Verification items for the finished model (mm, model axes). Face numbers are marked on the shaded views. A direction names the side the tool comes from. Coordinates: 2 decimals unless noted, no trailing zeros. Order: outer loops, then holes, each group sorted by start corner. A loop starts at its lowest first (then second) coordinate and runs counter-clockwise, first axis right, second up. Notation, with made-up numbers: (88, 0) -> (143, 0) arc R20 cw to (143, 29) -> close; hole circle Ø6 at (-38.5, 63.25). An arc over 180 degrees is marked (long way). Write each question's results on one line, items separated by ' | '. Start each with the question number.
(1) Cross-section at A-A on x = -2.5. Enter the section's corners in (y, z), and give its area (3 significant figures).
(2) Thickness scan on probe 1 along Y at (x, z) = (-3, -10); probe 2 along Y at (x, z) = (9.5, 3); probe 3 along Z at (x, y) = (1, 13.5). Record the ranges inside material, lowest first. Write a range as [from, to].
(3) Go/stop test with flat-tipped pins: pin 1 (7 mm diameter, centred on x = 0, y = 7.5, fed in from -Z); pin 2 (6 mm diameter, centred on x = 11, z = 12, fed in from +Y); pin 3 (3 mm diameter, centred on x = -8.01, z = 13.94, fed in from +Y); pin 4 (10 mm diameter, centred on y = 10.5, z = 3.19, fed in from +X) (1 decimal). Record where each tip stops, or that it passes through.
(4) Cross-section at C-C on x = -8.5. Enter the section's corners in (y, z).
(5) Set-up check for the marked faces 1, 2 and 3: record each of +Z, -Z, +X, -X, +Y, -Y from which the full face is reachable in a straight line by a thin tool's end or side.
(6) Draft check along Y on the marked faces 4, 5 and 6. Enter one of: +Y half, -Y half, draft (parallel to the pull), parting line (faces both ways), or undercut.
(7) Cross-section at B-B on y = 14. Enter the section's corners in (x, z).
(8) Cross-section at D-D on z = 0. Enter the section's corners in (x, y), and give its area (3 significant figures).
```python
from build123d import *

# Parameters (mm, degrees)
SKETCH1_W            = 27
SKETCH1_H            = 35
SKETCH1_R            = 1.113712744
SKETCH1_R_2          = 1.000106258
SKETCH1_R_3          = 1.174626552
SKETCH1_R_4          = 1.19920455
SKETCH1_W_2          = 8.3
SKETCH1_H_2          = 2.12
BOSS_EXTRUDE1_DEPTH  = 2
M2_CLEARANCE_HOLE2_D = 2.4
SKETCH13_W           = 27
SKETCH13_H           = 17
BOSS_EXTRUDE6_DEPTH  = 17
SKETCH14_R           = 6.4
CUT_EXTRUDE3_DEPTH   = 38.815687555


with BuildPart() as part:
    # Sketch1 → Boss-Extrude1 (new body)
    # profile 1 of 8: a face of its own
    with BuildSketch(Plane(origin=(0, 0, 0), x_dir=(1, 0, 0), z_dir=(0, 1, 0))):
        with Locations((0.988085162, -0.939800033)):
            Rectangle(SKETCH1_W, SKETCH1_H)
        Polygon((-10.011914838, -15.939800033), (-10.011914838, 14.060199967), (11.988085162, 14.060199967), (11.988085162, -15.939800033), (5.138085162, -15.939800033), (5.138085162, -18.059800033), (-3.161914838, -18.059800033), (-3.161914838, -15.939800033), align=None, mode=Mode.SUBTRACT)
    # profile 2 of 8: a face of its own
    with BuildSketch(Plane(origin=(0, 0, 0), x_dir=(1, 0, 0), z_dir=(0, 1, 0))):
        Polygon((11.988085162, 14.060199967), (-10.011914838, 14.060199967), (-10.011914838, -15.939800033), (-3.161914838, -15.939800033), (-3.161914838, -13.819800033), (5.138085162, -13.819800033), (5.138085162, -15.939800033), (11.988085162, -15.939800033), align=None)
        with Locations((-8.011914838, -13.939800033)):
            Circle(SKETCH1_R, mode=Mode.SUBTRACT)
        with Locations((9.988085162, -14.291814947)):
            Circle(SKETCH1_R_2, mode=Mode.SUBTRACT)
        with Locations((-8.011914838, 7.560199967)):
            Circle(SKETCH1_R_3, mode=Mode.SUBTRACT)
        with Locations((9.988085162, 7.560199967)):
            Circle(SKETCH1_R_4, mode=Mode.SUBTRACT)
    # profile 3 of 8: a face of its own
    with BuildSketch(Plane(origin=(0, 0, 0), x_dir=(1, 0, 0), z_dir=(0, 1, 0))):
        with Locations((-8.011914838, 7.560199967)):
            Circle(SKETCH1_R_3)
    # profile 4 of 8: a face of its own
    with BuildSketch(Plane(origin=(0, 0, 0), x_dir=(1, 0, 0), z_dir=(0, 1, 0))):
        with Locations((9.988085162, 7.560199967)):
            Circle(SKETCH1_R_4)
    # profile 5 of 8: a face of its own
    with BuildSketch(Plane(origin=(0, 0, 0), x_dir=(1, 0, 0), z_dir=(0, 1, 0))):
        with Locations((9.988085162, -14.291814947)):
            Circle(SKETCH1_R_2)
    # profile 6 of 8: a face of its own
    with BuildSketch(Plane(origin=(0, 0, 0), x_dir=(1, 0, 0), z_dir=(0, 1, 0))):
        with Locations((0.988085162, -16.999800033)):
            Rectangle(SKETCH1_W_2, SKETCH1_H_2)
    # profile 7 of 8: a face of its own
    with BuildSketch(Plane(origin=(0, 0, 0), x_dir=(1, 0, 0), z_dir=(0, 1, 0))):
        with Locations((0.988085162, -14.879800033)):
            Rectangle(SKETCH1_W_2, SKETCH1_H_2)
    # profile 8 of 8: a face of its own
    with BuildSketch(Plane(origin=(0, 0, 0), x_dir=(1, 0, 0), z_dir=(0, 1, 0))):
        with Locations((-8.011914838, -13.939800033)):
            Circle(SKETCH1_R)
    extrude(amount=BOSS_EXTRUDE1_DEPTH)

    # M2 Clearance Hole2 (through all)
    with Locations(Plane(origin=(0, 2, 0), x_dir=(1, 0, 0), z_dir=(0, 1, 0))):
        with Locations((-8.011914838, 7.560199967), (9.988085162, 7.560199967), (-8.011914838, -13.939800033), (9.988085162, -14.291814947)):
            Hole(M2_CLEARANCE_HOLE2_D / 2)

    # Sketch13 → Boss-Extrude6 (add)
    with BuildSketch(Plane(origin=(0, 2, 0), x_dir=(1, 0, 0), z_dir=(0, 1, 0))):
        with Locations((0.988085162, -3.189800033)):
            Rectangle(SKETCH13_W, SKETCH13_H)
    extrude(amount=BOSS_EXTRUDE6_DEPTH)

    # Sketch14 → Cut-Extrude3 (cut, through all)
    with BuildSketch(Plane(origin=(14.488085162, 0, 0), x_dir=(0, 0, -1), z_dir=(1, 0, 0))):
        with Locations((-3.189800033, 10.5)):
            Circle(SKETCH14_R)
        with BuildLine():
            Line((5.310199967, 19), (-3.189800009, 19))
            ThreePointArc((-3.189800009, 19), (2.820607616, 16.510407631), (5.310199967, 10.5))
            Line((5.310199967, 10.5), (5.310199967, 19))
        make_face()
        with BuildLine():
            Line((-3.189800009, 19), (-11.689800033, 19))
            Line((-11.689800033, 19), (-11.689800033, 10.50000002))
            ThreePointArc((-11.689800033, 10.50000002), (-9.200207658, 16.510407656), (-3.189800009, 19))
        make_face()
    extrude(amount=-CUT_EXTRUDE3_DEPTH, mode=Mode.SUBTRACT)


solid = part.part
```
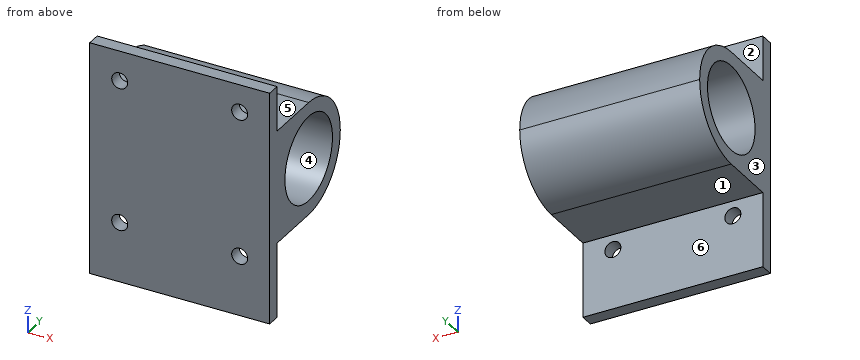
Results are:
1) outline: (0, -16.56) -> (2, -16.56) -> (2, -5.31) -> (10.5, -5.31) arc R8.5 ccw to (10.5, 11.69) -> (2, 11.69) -> (2, 18.44) -> (0, 18.44) -> close; hole circle Ø12.8 at (10.5, 3.19) | area: 199 mm2
2) probe 1: y = [0, 2] | probe 2: y = [0, 4.1], [16.9, 19] | probe 3: z = [-4.76, -2.46], [8.84, 11.14]
3) pin 1: stops at z = -5.31 | pin 2: stops at y = 16.7 | pin 3: stops at y = 2 | pin 4: passes through
4) outline: (0, -16.56) -> (2, -16.56) -> (2, -8.66) -> (0, -8.66) -> close; (0, -6.46) -> (2, -6.46) -> (2, -5.31) -> (10.5, -5.31) arc R8.5 ccw to (10.5, 11.69) -> (2, 11.69) -> (2, 12.84) -> (0, 12.84) -> close; (0, 15.04) -> (2, 15.04) -> (2, 18.44) -> (0, 18.44) -> close; hole circle Ø12.8 at (10.5, 3.19)
5) face 1: -Z, +X, -X, +Y | face 2: +Z, +X, -X, +Y | face 3: +Z, -Z, -X, +Y, -Y
6) face 4: undercut | face 5: draft | face 6: +Y half
7) outline: (-12.51, -4.56) -> (14.49, -4.56) -> (14.49, -2.17) -> (-12.51, -2.17) -> close; (-12.51, 8.55) -> (14.49, 8.55) -> (14.49, 10.94) -> (-12.51, 10.94) -> close
8) outline: (-12.51, 0) -> (14.49, 0) -> (14.49, 4.95) -> (-12.51, 4.95) -> close; (-12.51, 16.05) -> (14.49, 16.05) -> (14.49, 18.38) -> (-12.51, 18.38) -> close | area: 197 mm2
